Here's the drawing with two shaded views (mm, measured from the low corner). I have some questions. A direction names the side the tool comes from. Give positions to 0.01 mm unless a question says otherwise; leave off trailing zeros. Write each loop counter-clockwise with the first axis right and the second up, starting at its lowest first coordinate (ties: lowest second). Pieces come first, ordered by that corner, then holes. Notation, with made-up numbers: (35.25, 42.25) -> (67.25, 42.25) arc R15 ccw to (67.25, 68.25) -> close; hole circle Ø8 at (63, 75). An arc over 180 degrees is marked (long way). One line per item, written item: value.
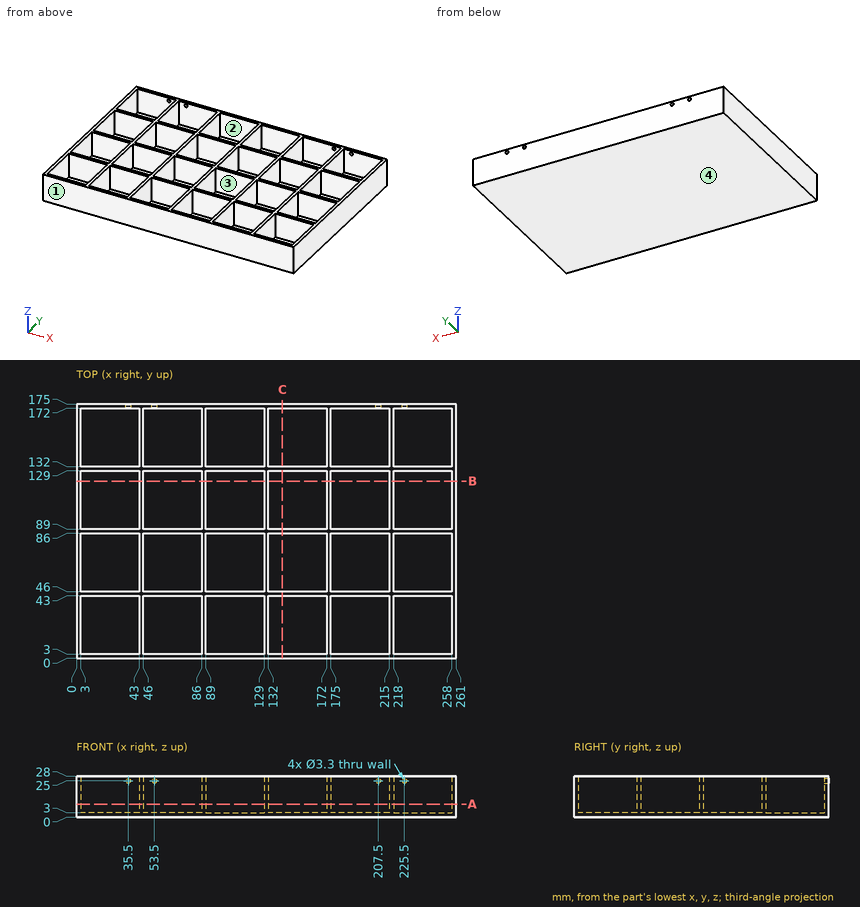
1) I need wall thicknesses on L1, parallel to Y at x = 28.5, z = 9.5; L2, parallel to X at y = 173.7, z = 25; L3, parallel to Z at x = 207.5, y = 174.15. Which ranges of each line are inside material? Lowest first, please.
Answer list:
L1: y = 0 to 3, 43 to 46, 86 to 89, 129 to 132, 172 to 175
L2: x = 0 to 33.85, 37.15 to 51.85, 55.15 to 205.85, 209.15 to 223.85, 227.15 to 261
L3: z = 0 to 23.35, 26.65 to 28
2) If we section it at A-A (z = 9): State how many separate pieces and enclosed holes the cut face has, and give its area (4 significant figures).
Answer list:
separate pieces: 1
enclosed holes: 24
area: 7,275 mm^2
3) If we section it at B-B (y = 122): Write out the boundary of the cut face in (x, z), and give its area (3 significant figures).
Answer list:
outline: (0, 0) -> (261, 0) -> (261, 28) -> (258, 28) -> (258, 3) -> (218, 3) -> (218, 28) -> (215, 28) -> (215, 3) -> (175, 3) -> (175, 28) -> (172, 28) -> (172, 3) -> (132, 3) -> (132, 28) -> (129, 28) -> (129, 3) -> (89, 3) -> (89, 28) -> (86, 28) -> (86, 3) -> (46, 3) -> (46, 28) -> (43, 28) -> (43, 3) -> (3, 3) -> (3, 28) -> (0, 28) -> close
area: 1,310 mm^2
4) We'd pull the mould along X, two halves only. Please class the marked faces 1 and 2: released by +X, released by -X, zero draft, split by the parting line, or undercut.
Answer list:
face 1: zero draft
face 2: undercut
5) For the marked faces 3 and 4, which set-ups out of +Z, -Z, +X, -X, +Y, -Y let a thin tool reach every point of the face, with its end or its side?
Answer list:
face 3: +Z
face 4: -Z, +X, -X, +Y, -Y
6) If we section it at C-C (x = 141.5): Write out the boundary of the cut face in (y, z).
Answer list:
outline: (0, 0) -> (175, 0) -> (175, 28) -> (172, 28) -> (172, 3) -> (132, 3) -> (132, 28) -> (129, 28) -> (129, 3) -> (89, 3) -> (89, 28) -> (86, 28) -> (86, 3) -> (46, 3) -> (46, 28) -> (43, 28) -> (43, 3) -> (3, 3) -> (3, 28) -> (0, 28) -> close
